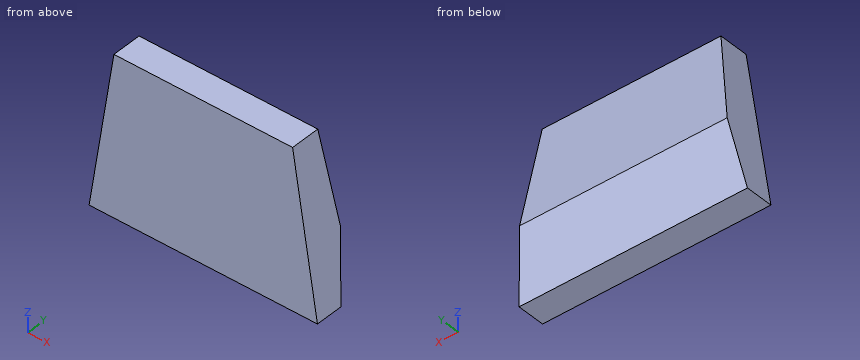
```python
from build123d import *

# Parameters (mm, degrees)
BOSS_EXTRUDE1_DEPTH = 50.8
CHAMFER1_SIZE       = 12.7
CHAMFER1_SIZE2      = 120.832428569
CHAMFER2_SIZE       = 86.430334931
CHAMFER2_SIZE_2     = 15.24


with BuildPart() as part:
    # Sketch1 → Boss-Extrude1 (new body)
    with BuildSketch(Plane(origin=(0, 0, 0), x_dir=(1, 0, 0), z_dir=(0, 1, 0))):
        Polygon((0, 0), (292.1, 0), (260.35, -203.2), (31.75, -203.2), align=None)
    extrude(amount=BOSS_EXTRUDE1_DEPTH)

    # Chamfer1
    chamfer1_edges = [part.edges().sort_by_distance(p)[0] for p in [
        (146.05, 50.8, 203.2),
    ]]
    chamfer1_side = [part.faces().sort_by_distance(p)[0] for p in [
        (146.05, 25.4, 203.2),
    ]]
    chamfer(chamfer1_edges, length=CHAMFER1_SIZE, length2=CHAMFER1_SIZE2, reference=chamfer1_side[0])

    # Chamfer2
    # the kernel refuses this chamfer: 86.430334931, 15.24 mm, written as the material it takes off along each edge
    with BuildSketch(Plane(origin=(-224.592578506, 50.8, 0), x_dir=(0, 0.006682531656101609, 0.9999776716360547), z_dir=(1, 0, 0))) as chamfer2_piece_1:
        Polygon((CHAMFER2_SIZE * 0.999977671636, CHAMFER2_SIZE * 0.0066825316561), (-CHAMFER2_SIZE_2 * 0.0066825316561, CHAMFER2_SIZE_2 * 0.999977671636), (0, 0), align=None)
    extrude(amount=741.285157012, mode=Mode.SUBTRACT)


solid = part.part
```
Input: part model. Units: mm. Frame: model coordinates. Coordinates: 2 decimals unless noted, no trailing zeros. Loops run counter-clockwise (first coordinate to the right, second up) from the corner with the lowest first, then second, coordinate; pieces in that order, holes last. Notation, with made-up numbers: (33.25, 63.25) - (51.25, 63.25) arc R17 cw to (51.25, 81.25) - close; hole circle Ø9 at (14, -31). An arc over 180 degrees is marked (long way). Answer in a Markdown table with one row per item.
(1) Cut plane A-A on x = 75. Output: boundary loops of the cut face in (y, z).
Model answer:
| item | result |
|---|---|
| outline | (0, 0) - (35.56, 0) - (50.53, 84.91) - (38.1, 203.2) - (0, 203.2) - close |
(2) Cut plane C-C on z = 90. Output: boundary loops of the cut face in (x, y), plus the area to 3 significant figures.
Model answer:
| item | result |
|---|---|
| outline | (14.06, 0) - (278.04, 0) - (278.04, 50) - (14.06, 50) - close |
| area | 13,200 mm² |
(3) Material intervals for L1, parallel to X at y = 37, z = 82; L2, parallel to Y at x = 75, z = 87; L3, parallel to X at y = 5, z = 166, sorted ascending. Write a range as from..to.
Model answer:
| item | result |
|---|---|
| L1 | x = 12.81..279.29 |
| L2 | y = 0..50.31 |
| L3 | x = 25.94..266.16 |
(4) Cut plane B-B on y = 23.5. Output: boundary loops of the cut face in (x, z), plus the area to 3 significant figures.
Model answer:
| item | result |
|---|---|
| outline | (0, 0) - (292.1, 0) - (260.35, 203.2) - (31.75, 203.2) - close |
| area | 52,900 mm² |
(5) Pin query (flat end, axial travel): P1, Ø8, axis at y = 33.5, z = 81, coming from the +X side; P2, Ø12, axis at x = 70.5, z = 124.5, coming from the +Y side; P3, Ø1, axis at y = 24.5, z = 68.5, coming from the -X side (3 decimals). Return the tip coordinate at first contact, or that it passes through.
Model answer:
| item | result |
|---|---|
| P1 | stops at x = 280.07 |
| P2 | stops at y = 47 |
| P3 | stops at x = 10.625 |
